from build123d import *

# Parameters (mm, degrees)
CHAMFER1_SIZE      = 0.25
FILLET1_R          = 0.2
CUT_EXTRUDE1_DEPTH = 2
FILLET2_R          = 0.1


with BuildPart() as part:
    # Sketch1 → Revolve1 (revolve)
    with BuildSketch(Plane.XY):
        Polygon((0, -9), (-1.5, -9), (-1.5, -3), (-2.75, -3), (-2.75, 0), (0, 0), align=None)
    revolve(axis=Axis((0, 0, 0), (0, -1, 0)))

    # Chamfer1
    chamfer1_edges = [part.edges().sort_by_distance(p)[0] for p in [
        (1.5, -3, 0),
        (1.5, -9, 0),
    ]]
    chamfer(chamfer1_edges, length=CHAMFER1_SIZE)

    # Fillet1
    fillet1_edges = [part.edges().sort_by_distance(p)[0] for p in [
        (2.75, 0, 0),
    ]]
    fillet(fillet1_edges, radius=FILLET1_R)

    # Sketch2 → Cut-Extrude1 (cut)
    with BuildSketch(Plane(origin=(0, 0, 0), x_dir=(1, 0, 0), z_dir=(0, 1, 0))):
        Polygon((0, 1.443375673), (-1.25, 0.721687836), (-1.25, -0.721687836), (0, -1.443375673), (1.25, -0.721687836), (1.25, 0.721687836), align=None)
    extrude(amount=-CUT_EXTRUDE1_DEPTH, mode=Mode.SUBTRACT)

    # Fillet2
    fillet2_edges = [part.edges().sort_by_distance(p)[0] for p in [
        (0.625, -2, -1.082531755),
        (1.25, -2, 0),
        (0.625, -2, 1.082531755),
        (-0.625, -2, 1.082531755),
        (-1.25, -2, 0),
        (-0.625, -2, -1.082531755),
        (0.625, 0, -1.082531755),
        (-0.625, 0, -1.082531755),
        (-1.25, 0, 0),
        (-0.625, 0, 1.082531755),
        (0.625, 0, 1.082531755),
        (1.25, 0, 0),
    ]]
    fillet(fillet2_edges, radius=FILLET2_R)


solid = part.part
Design review of the part built by this model. Coordinates are the model's own, in mm. A direction names the side the tool comes from. Give positions to 0.01 mm unless a question says otherwise; leave off trailing zeros. Loops run counter-clockwise (first coordinate to the right, second up) from the corner with the lowest first, then second, coordinate; pieces in that order, holes last. Notation, with made-up numbers: M 27.25,53 L 86.25,53 A18 cw 86.25,65 Z; hole C 13.5,-5.75 d9. An arc over 180 degrees is marked long. Write item = value, one per line.
Q1. Draft analysis for pull direction X (two halves, no side actions). For faces 1 (the cylindrical face through (0.596, -1.58, 2.685)), 2 (the flat face through (0, -9, 0)), 3 (the flat face through (0.616, -0.987, 1.088)), state which applies: +X half, -X half, draft (parallel to the pull), parting line (faces both ways), or undercut.
Output values:
face_1 = parting line
face_2 = draft
face_3 = undercut
Q2. To check wall thickness, follow line 1 (Z direction, x = 0.4, y = -7); line 2 (Y direction, x = 0.15, z = -2.35); line 3 (Z direction, x = 0.3, y = -1.5). State the ranges of each line that lie inside material, in increasing order. Write a range as [from, to].
Output values:
line_1 = [-1.45, 1.45]
line_2 = [-3, 0]
line_3 = [-2.73, -1.27], [1.27, 2.73]
Q3. We need section B-B (z = 0). Give the boundary of the cut face in (x, y), plus the area to 3 significant figures.
Output values:
outline = M -2.75,-3 L -1.75,-3 L -1.5,-3.25 L -1.5,-8.75 L -1.25,-9 L 1.25,-9 L 1.5,-8.75 L 1.5,-3.25 L 1.75,-3 L 2.75,-3 L 2.75,-0.2 A0.2 ccw 2.55,0 L 1.35,0 A0.1 ccw 1.25,-0.1 L 1.25,-1.9 A0.1 cw 1.15,-2 L -1.15,-2 A0.1 cw -1.25,-1.9 L -1.25,-0.1 A0.1 ccw -1.35,0 L -2.55,0 A0.2 ccw -2.75,-0.2 Z
area = 29.5 mm^2
Q4. We need section D-D (y = -2.75). Give the boundary of the cut face in (x, z).
Output values:
outline = C 0,0 d5.5
Q5. We need section C-C (y = -4.5). Give the boundary of the cut face in (x, z), plus the area to 3 significant figures.
Output values:
outline = C 0,0 d3
area = 7.07 mm^2
Q6. Insertion check: pin 1 (0.7 mm diameter, centred on x = 0, z = -0.5, fed in from +Y); pin 2 (1 mm diameter, centred on y = -2, z = -1, fed in from -X); pin 3 (1 mm diameter, centred on y = -3, z = 0.5, fed in from +X). Each pin has a flat end and moves straight along its axis. Give the tip position at first contact, or say it passes through.
Output values:
pin_1 = -2
pin_2 = -2.7
pin_3 = 2.75
Q7. We need section A-A (y = -1.5). Give the boundary of the cut face in (x, z).
Output values:
outline = C 0,0 d5.5; hole M -1.25,-0.72 L 0,-1.44 L 1.25,-0.72 L 1.25,0.72 L 0,1.44 L -1.25,0.72 Z
Q8. For faces 4 (the flat face through (-1.1, 0, 1.1)), 5 (the flat face through (-0.63, -0.99, 1.08)), 6 (the cylindrical face through (1.5, -5.96, -0.07)), list the 3-axis set-ups (+Z, -Z, +X, -X, +Y, -Y) from which the entire face can be reached by the end or side of a thin tool; tool diameter is ignored.
Output values:
face_4 = +Z, -Z, +X, -X, +Y
face_5 = +Y
face_6 = -Y
